Model file for the job. Use its own axes, mm. Face numbers are marked on the shaded views. A direction names the side the tool comes from. Give positions to 0.01 mm unless a question says otherwise; leave off trailing zeros. Order: outer loops, then holes, each group sorted by start corner. A loop starts at its lowest first (then second) coordinate and runs counter-clockwise, first axis right, second up. Notation, with made-up numbers: (85.5, 2) -> (108.5, 2) arc R15 cw to (108.5, 18) -> close; hole circle Ø11 at (43, -3). An arc over 180 degrees is marked (long way). Answer in a Markdown table with one row per item. Add a question column.
from build123d import *

# Parameters (mm, degrees)
F0_R        = 7.9375
F1_DEPTH    = 38.1
F2_T1_DEPTH = 85.725
F3_T1_DEPTH = 38.1


# Not quite as in the source:
# - a fillet or chamfer that OpenCascade refuses, or shapes differently, is made with other operations: its cross-section is extruded or revolved along the edge and cut away or added
# - a length typed as a fraction of an inch, garbled in the dataset ("3 / 203.2 mm" for 3/8 in), is restored


with BuildPart() as f1:
    # F0 (on Top) → F1 (new body)
    with BuildSketch(Plane.XY):
        with BuildLine():
            Line((16.4977839421, -9.525), (177.8, -9.525))
            Line((177.8, -9.525), (177.8, 9.525))
            Line((177.8, 9.525), (16.4977839421, 9.525))
            ThreePointArc((16.4977839421, 9.525), (0, 19.05), (-16.4977839421, 9.525))
            Line((-16.4977839421, 9.525), (-177.8, 9.525))
            Line((-177.8, 9.525), (-177.8, -9.525))
            Line((-177.8, -9.525), (-16.4977839421, -9.525))
            ThreePointArc((-16.4977839421, -9.525), (0, -19.05), (16.4977839421, -9.525))
        make_face()
        Circle(F0_R, mode=Mode.SUBTRACT)
        Circle(F0_R)
    extrude(amount=F1_DEPTH)

    # F2: fillet of radius 9.525 on 4 edges, made by hand

    # F2_s2 → F2_t1 (cut)
    with BuildSketch(Plane.XY.offset(-23.8125)):
        with BuildLine():
            add(Edge.make_bspline(
                [(-177.8, 0), (-177.8, -9.525), (-168.275, -9.525)],
                knots=[0, 0, 0, 1, 1, 1], degree=2, weights=[1, 1.8571428571, 1]))
            Line((-168.275, -9.525), (-177.8, -9.525))
            Line((-177.8, -9.525), (-177.8, 0))
        make_face()
        with BuildLine():
            add(Edge.make_bspline(
                [(-168.275, 9.525), (-177.8, 9.525), (-177.8, 0)],
                knots=[0, 0, 0, 1, 1, 1], degree=2, weights=[1, 1.8571428571, 1]))
            Line((-177.8, 0), (-177.8, 9.525))
            Line((-177.8, 9.525), (-168.275, 9.525))
        make_face()
        with BuildLine():
            add(Edge.make_bspline(
                [(177.8, 0), (177.8, 9.525), (168.275, 9.525)],
                knots=[0, 0, 0, 1, 1, 1], degree=2, weights=[1, 1.8571428571, 1]))
            Line((168.275, 9.525), (177.8, 9.525))
            Line((177.8, 9.525), (177.8, 0))
        make_face()
        with BuildLine():
            add(Edge.make_bspline(
                [(168.275, -9.525), (177.8, -9.525), (177.8, 0)],
                knots=[0, 0, 0, 1, 1, 1], degree=2, weights=[1, 1.8571428571, 1]))
            Line((177.8, 0), (177.8, -9.525))
            Line((177.8, -9.525), (168.275, -9.525))
        make_face()
    extrude(amount=F2_T1_DEPTH, mode=Mode.SUBTRACT)

    # F3: fillet of radius 64.0333905996 on 4 edges, made by hand

    # F3_s2 → F3_t1 (join)
    with BuildSketch(Plane.XY):
        with BuildLine():
            add(Edge.make_bspline(
                [(8.8566007427, 16.8660346046), (22.8364726227, 9.525), (38.6265836688, 9.525)],
                knots=[0, 0, 0, 1, 1, 1], degree=2, weights=[1, 1.8571428571, 1]))
            Line((38.6265836688, 9.525), (16.4977839421, 9.525))
            ThreePointArc((16.4977839421, 9.525), (13.1978749408, 13.737488746), (8.8566007427, 16.8660346046))
        make_face()
        with BuildLine():
            add(Edge.make_bspline(
                [(-38.6265836688, 9.525), (-22.8364726227, 9.525), (-8.8566007427, 16.8660346046)],
                knots=[0, 0, 0, 1, 1, 1], degree=2, weights=[1, 1.8571428571, 1]))
            ThreePointArc((-8.8566007427, 16.8660346046), (-13.1978749408, 13.737488746), (-16.4977839421, 9.525))
            Line((-16.4977839421, 9.525), (-38.6265836688, 9.525))
        make_face()
        with BuildLine():
            add(Edge.make_bspline(
                [(-8.8566007427, -16.8660346046), (-22.8364726227, -9.525), (-38.6265836688, -9.525)],
                knots=[0, 0, 0, 1, 1, 1], degree=2, weights=[1, 1.8571428571, 1]))
            Line((-38.6265836688, -9.525), (-16.4977839421, -9.525))
            ThreePointArc((-16.4977839421, -9.525), (-13.1978749408, -13.737488746), (-8.8566007427, -16.8660346046))
        make_face()
        with BuildLine():
            add(Edge.make_bspline(
                [(8.8566007427, -16.8660346046), (22.8364726227, -9.525), (38.6265836688, -9.525)],
                knots=[0, 0, 0, 1, 1, 1], degree=2, weights=[1, 1.8571428571, 1]))
            Line((38.6265836688, -9.525), (16.4977839421, -9.525))
            ThreePointArc((16.4977839421, -9.525), (13.1978749408, -13.737488746), (8.8566007427, -16.8660346046))
        make_face()
    extrude(amount=F3_T1_DEPTH)


solid = f1.part
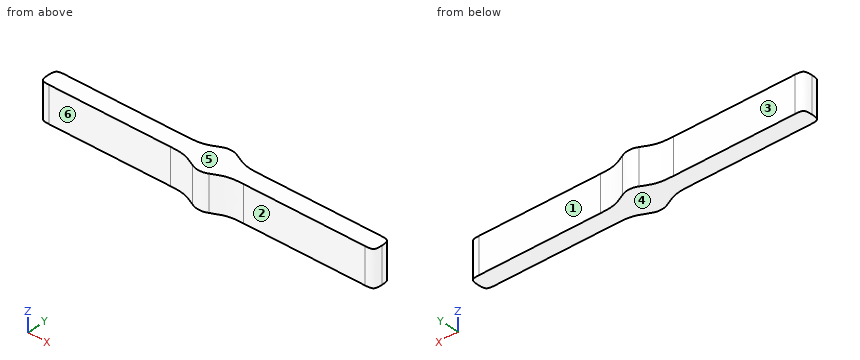
Item 1: Which spindle directions (+Z, -Z, +X, -X, +Y, -Y) get a long thin tool onto all of the face, cutting with end or side? Do the marked faces 1, 2 and 3. Say none if no direction does.
Item 2: Two-plate mould, pull along Z, no slides. Class the marked faces 4, 5 and 6: pulls with the +Z half, pulls with the -Z half, needs draft (parallel to the pull), parting line crosses it, or undercut.
Item 3: Wall check: line 1 (Y direction, x = 94.5, z = 20) (3 decimals); line 2 (X direction, y = 2, z = 6); line 3 (X direction, y = -16.5, z = 22). Give the ranges that are in metal, low to high.
Item 4: Pin check, flat tips, straight feed: pin 1 Ø10 at (x, z) = (-2, 14.5) entering from -Y; pin 2 Ø19 at (x, z) = (102.5, 15) entering from +Y (3 decimals); pin 3 Ø19 at (x, z) = (-87, 23.5) entering from -Y (3 decimals). Stop position of each tip, or through.
Item 5: Saw through at A-A on x = -116. List the corners of the cut face in (y, z) (3 decimals).
Evaluation:
| question | item | result |
|---|---|---|
| 1 | face 1 | +Z, -Z, +X, +Y |
| 1 | face 2 | +Z, -Z, +X, -Y |
| 1 | face 3 | +Z, -Z, -X, +Y |
| 2 | face 4 | pulls with the -Z half |
| 2 | face 5 | pulls with the +Z half |
| 2 | face 6 | needs draft |
| 3 | line 1 | y = -9.525 to 9.525 |
| 3 | line 2 | x = -177.76 to 177.76 |
| 3 | line 3 | x = -9.56 to 9.56 |
| 4 | pin 1 | stops at y = -19.05 |
| 4 | pin 2 | stops at y = 9.525 |
| 4 | pin 3 | stops at y = -9.525 |
| 5 | outline | (-9.525, 0) -> (9.525, 0) -> (9.525, 38.1) -> (-9.525, 38.1) -> close |
